Build history of the part. All positions in model axes, mm. A direction names the side the tool comes from. Round coordinates to 2 decimals unless told otherwise and drop trailing zeros. Loops run counter-clockwise (first coordinate to the right, second up) from the corner with the lowest first, then second, coordinate; pieces in that order, holes last. Notation, with made-up numbers: M -33,-20.5 L 10,-20.5 A21 ccw 10,10.5 Z; hole C 14,49 d1. An arc over 180 degrees is marked long. One line per item, written item: value.
```python
from build123d import *

# Parameters (mm, degrees)
CROQUIS1_W              = 8
CROQUIS1_H              = 3
SALIENTE_EXTRUIR1_DEPTH = 3
REDONDEO1_R             = 2


with BuildPart() as part:
    # Croquis1 → Saliente-Extruir1 (new body)
    with BuildSketch(Plane.XY):
        with BuildLine():
            Line((-12.5, 0), (-7.703315155, -2.870856056))
            ThreePointArc((-7.703315155, -2.870856056), (0, -5), (7.703315155, -2.870856056))
            Line((7.703315155, -2.870856056), (12.5, 0))
            Line((12.5, 0), (-12.5, 0))
        make_face()
        with Locations((-8.5, 1.5)):
            Rectangle(CROQUIS1_W, CROQUIS1_H)
        with Locations((8.5, 1.5)):
            Rectangle(CROQUIS1_W, CROQUIS1_H)
    extrude(amount=SALIENTE_EXTRUIR1_DEPTH)

    # Redondeo1
    redondeo1_edges = [part.edges().sort_by_distance(p)[0] for p in [
        (-12.5, 0, 1.5),
        (12.5, 0, 1.5),
    ]]
    fillet(redondeo1_edges, radius=REDONDEO1_R)


solid = part.part
```
Item 1: Wall check: line 1 along X through (y, z) = (1.75, 1); line 2 along X through (y, z) = (0.5, 0.3); line 3 along Y through (x, z) = (-5.75, 0.3). Give the ranges that are in metal, low to high.
Check values:
line 1: x = -12.5 to -4.5, 4.5 to 12.5
line 2: x = -12.4 to -4.5, 4.5 to 12.4
line 3: y = -3.85 to 3
Item 2: Pull direction X, two halves, no side cores. Call faces 3 (the face through (0, 0, 1)), 4 (the face through (-12.5, 2, 1)), 5 (the face through (9.59, -1.74, 1.48)): pulls with the +X half, pulls with the -X half, needs draft (parallel to the pull), parting line crosses it, or undercut.
Check values:
face 3: undercut
face 4: pulls with the -X half
face 5: pulls with the +X half
Item 3: Slice it at B-B, the plane y = 0.25. Give the cut face in (x, z), and give its area (3 significant figures).
Check values:
outline: M -12.29,0 L -4.5,0 L -4.5,3 L -12.29,3 Z; M 4.5,0 L 12.29,0 L 12.29,3 L 4.5,3 Z
area: 46.8 mm2
Item 4: Which spindle directions (+Z, -Z, +X, -X, +Y, -Y) get a long thin tool onto all of the face, cutting with end or side? Do faces 1 (the face through (-4.5, 1, 1)), 2 (the face through (-9, 3, 1)). Say none if no direction does.
Check values:
face 1: +Z, -Z, +Y
face 2: +Z, -Z, +X, -X, +Y
Item 5: Slice it at D-D, the plane y = -1. Give the cut face in (x, z), and give its area (3 significant figures).
Check values:
outline: M -10.83,0 L 10.83,0 L 10.83,3 L -10.83,3 Z
area: 65.0 mm2
Item 6: Slice it at A-A, the plane z = 2.55. Give the cut face in (x, y).
Check values:
outline: M -12.5,1.13 A2 ccw -11.53,-0.58 L -7.7,-2.87 A15 ccw 7.7,-2.87 L 11.53,-0.58 A2 ccw 12.5,1.13 L 12.5,3 L 4.5,3 L 4.5,0 L -4.5,0 L -4.5,3 L -12.5,3 Z
Item 7: Drop a flat-ended pin along its axis: P1, Ø0.9, axis at x = 1, z = 1.5, coming from the +Y side. Give the stop position or say it passes through.
Check values:
P1: stops at y = 0
Item 8: Slice it at C-C, the plane x = -2. Give the cut face in (y, z).
Check values:
outline: M -4.87,0 L 0,0 L 0,3 L -4.87,3 Z
